Part model, mm, in its own coordinate system. A direction names the side the tool comes from. Give positions to 0.01 mm unless a question says otherwise; leave off trailing zeros. Loops run counter-clockwise (first coordinate to the right, second up) from the corner with the lowest first, then second, coordinate; pieces in that order, holes last. Notation, with made-up numbers: (-13, -3) -> (5, -3) arc R6 ccw to (5, 5) -> close; hole circle Ø1 at (82.5, -7.5). An arc over 180 degrees is marked (long way). One line per question, with ' | ' between items.
```python
from build123d import *

# Parameters (mm, degrees)
BOSS_EXTRUDE1_DEPTH = 40
SKETCH2_R           = 60
BOSS_EXTRUDE2_DEPTH = 10
SKETCH3_R           = 58
CUT_EXTRUDE1_DEPTH  = 12
SKETCH5_R           = 68
CUT_EXTRUDE3_DEPTH  = 38
SKETCH7_W           = 152.426139127
SKETCH7_H           = 144.716969628
CUT_EXTRUDE4_DEPTH  = 10
CUT_EXTRUDE6_DEPTH  = 2


with BuildPart() as part:
    # Sketch1 → Boss-Extrude1 (new body)
    with BuildSketch(Plane(origin=(0, 0, 0), x_dir=(1, 0, 0), z_dir=(0, 1, 0))):
        with BuildLine():
            Line((-30, 70), (30, 70))
            ThreePointArc((30, 70), (58.284271247, 58.284271247), (70, 30))
            Line((70, 30), (70, -30))
            ThreePointArc((70, -30), (58.284271247, -58.284271247), (30, -70))
            Line((30, -70), (-30, -70))
            ThreePointArc((-30, -70), (-58.284271247, -58.284271247), (-70, -30))
            Line((-70, -30), (-70, 30))
            ThreePointArc((-70, 30), (-58.284271247, 58.284271247), (-30, 70))
        make_face()
    extrude(amount=-BOSS_EXTRUDE1_DEPTH)

    # Sketch2 → Boss-Extrude2 (add)
    with BuildSketch(Plane(origin=(0, 0, 0), x_dir=(1, 0, 0), z_dir=(0, 1, 0))):
        with Locations(Location((0, 0, 0), (0, 0, 270))):
            Circle(SKETCH2_R)
    extrude(amount=BOSS_EXTRUDE2_DEPTH)

    # Sketch3 → Cut-Extrude1 (cut)
    with BuildSketch(Plane(origin=(0, 10, 0), x_dir=(1, 0, 0), z_dir=(0, 1, 0))):
        with Locations(Location((0, 0, 0), (0, 0, 270))):
            Circle(SKETCH3_R)
    extrude(amount=-CUT_EXTRUDE1_DEPTH, mode=Mode.SUBTRACT)

    # Sketch5 → Cut-Extrude3 (cut)
    with BuildSketch(Plane.XZ.offset(40)):
        with Locations(Location((0, 0, 0), (0, 0, 270))):
            Circle(SKETCH5_R)
    extrude(amount=-CUT_EXTRUDE3_DEPTH, mode=Mode.SUBTRACT)

    # Sketch7 → Cut-Extrude4 (cut)
    with BuildSketch(Plane.XZ.offset(40)):
        with Locations((-0.48756258, -1.365678106)):
            Rectangle(SKETCH7_W, SKETCH7_H)
    extrude(amount=-CUT_EXTRUDE4_DEPTH, mode=Mode.SUBTRACT)

    # Sketch8 → Cut-Extrude6 (cut)
    with BuildSketch(Plane.XZ.offset(30)):
        with BuildLine():
            Line((68, 30), (68, -30))
            ThreePointArc((68, -30), (56.870057685, -56.870057685), (30, -68))
            Line((30, -68), (-30, -68))
            ThreePointArc((-30, -68), (-56.870057685, -56.870057685), (-68, -30))
            Line((-68, -30), (-68, 30))
            ThreePointArc((-68, 30), (-56.870057685, 56.870057685), (-30, 68))
            Line((-30, 68), (30, 68))
            ThreePointArc((30, 68), (56.870057685, 56.870057685), (68, 30))
        make_face()
    extrude(amount=-CUT_EXTRUDE6_DEPTH, mode=Mode.SUBTRACT)


solid = part.part
```
1) Saw through at B-B (z = -10). Give the cut face in (x, y).
Found:
outline: (-70, -30) -> (-68, -30) -> (-68, -28) -> (-67.26, -28) -> (-67.26, -2) -> (-57.13, -2) -> (-57.13, 10) -> (-59.16, 10) -> (-59.16, 0) -> (-70, 0) -> close; (57.13, -2) -> (67.26, -2) -> (67.26, -28) -> (68, -28) -> (68, -30) -> (70, -30) -> (70, 0) -> (59.16, 0) -> (59.16, 10) -> (57.13, 10) -> close
2) Saw through at C-C (x = -18.5). Give the cut face in (y, z), and give its area (3 significant figures).
Found:
outline: (-30, -70) -> (0, -70) -> (0, -57.08) -> (10, -57.08) -> (10, -54.97) -> (-2, -54.97) -> (-2, -65.44) -> (-28, -65.44) -> (-28, -68) -> (-30, -68) -> close; (-30, 68) -> (-28, 68) -> (-28, 65.44) -> (-2, 65.44) -> (-2, 54.97) -> (10, 54.97) -> (10, 57.08) -> (0, 57.08) -> (0, 70) -> (-30, 70) -> close | area: 348 mm2
3) Tool access for faces 1 (the cylindrical face through (58.594, -14.79, 57.972)), 2 (the flat face through (-49, -28, 49)), 3 (the flat face through (63, 0, -1)): list every direction of +Z, -Z, +X, -X, +Y, -Y with a clear straight run to the whole face (end or side of a thin tool).
Found:
face 1: +Z, +X, +Y, -Y | face 2: -Y | face 3: +Y
4) Pin check, flat tips, straight feed: P1, Ø4, axis at y = -8.5, z = -42, coming from the +X side; P2, Ø20.5, axis at x = 46.5, z = 44, coming from the -Y side; P3, Ø2, axis at x = 45, y = -9.5, coming from the +Z side. Stop position of each tip, or through.
Found:
P1: x = 68.73 | P2: y = -28 | P3: z = 67.47
5) Drill centre lines: line 1 (Z direction, x = 0, y = -21.75); line 2 (Y direction, x = -52, z = -47). Where is each one in solid material? Low to high.
Found:
line 1: -70 to -68, 68 to 70 | line 2: -28 to 0
6) Saw through at A-A (y = -15). Give the cut face in (x, z), and give its area (3 significant figures).
Found:
outline: (-70, -30) arc R40 ccw to (-30, -70) -> (30, -70) arc R40 ccw to (70, -30) -> (70, 30) arc R40 ccw to (30, 70) -> (-30, 70) arc R40 ccw to (-70, 30) -> close; hole circle Ø136 at (0, 0) | area: 3,700 mm2
